Part model, mm, in its own coordinate system. Face numbers are marked on the shaded views. Coordinates: 2 decimals unless noted, no trailing zeros. Loops run counter-clockwise (first coordinate to the right, second up) from the corner with the lowest first, then second, coordinate; pieces in that order, holes last. Notation, with made-up numbers: (69, 88.25) -> (111, 88.25) arc R23 ccw to (111, 100.25) -> close; hole circle Ø2 at (28, -35). An arc over 180 degrees is marked (long way). One line per question, with ' | ' between items. Start each with the question number.
1) Cut at D-D (x = 4.5). List the corners of the cut face in (y, z), plus the area to 3 significant figures.
2) Cut at C-C (x = 28). List the corners of the cut face in (y, z), plus the area to 3 significant figures.
3) Cut at A-A (z = 15). List the corners of the cut face in (x, y).
4) Two-plate mould, pull along X, no slides. Class the marked faces 1, 2, 3 and 4: released by +X, released by -X, zero draft, split by the parting line, or undercut.
5) Cut at B-B (y = -53). List the corners of the cut face in (x, z), plus the area to 3 significant figures.
6) Drop flat-ended pins along their axis: pin 1 (4 mm diameter, centred on x = -6, y = -44.5, fed in from +Z); pin 2 (5 mm diameter, centred on y = -6.5, z = 12, fed in from +X); pin 3 (6 mm diameter, centred on x = -27, y = -35.5, fed in from +Z). Give the stop position or say it passes through.
7) Probe L1, parallel to Y at x = 7, z = 9.75; L2, parallel to Y at x = -9, z = 6.75; L3, parallel to Y at x = -2, z = 18. List the from-to ranges inside material, lowest first. Write a range as from..to.
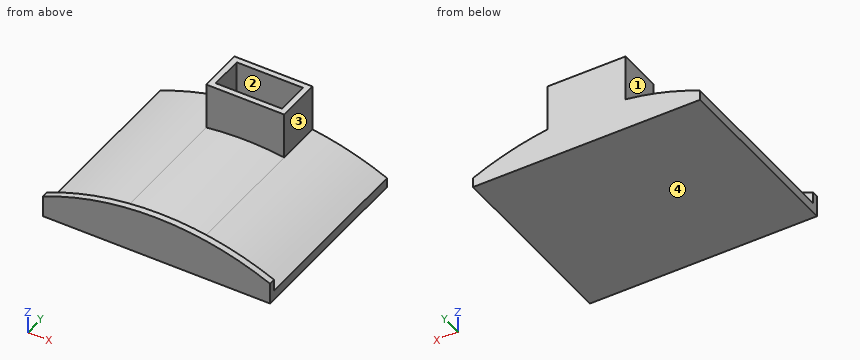
from build123d import *

# Parameters (mm, degrees)
F1_DEPTH = 58
F2_DEPTH = 14
F4_DEPTH = 2
F5_W     = 20.4
F5_H     = 10.4
F6_DEPTH = 22


with BuildPart() as f1:
    # F0 (on Front) → F1 (new body)
    with BuildSketch(Plane.XZ):
        with BuildLine():
            Line((35, -3), (35, 0))
            ThreePointArc((35, 0), (23.7368009031, 4.158739596), (12, 6.6890110215))
            Line((12, 6.6890110215), (12, 0))
            Line((12, 0), (-12, 0))
            Line((-12, 0), (-12, 6.6890110215))
            ThreePointArc((-12, 6.6890110215), (-23.7368009031, 4.158739596), (-35, 0))
            Line((-35, 0), (-35, -3))
            Line((-35, -3), (35, -3))
        make_face()
        with BuildLine():
            Line((12, 0), (12, 6.6890110215))
            ThreePointArc((12, 6.6890110215), (0, 7.5403330759), (-12, 6.6890110215))
            Line((-12, 6.6890110215), (-12, 0))
            Line((-12, 0), (12, 0))
        make_face()
    extrude(amount=F1_DEPTH)

    # F0 (on Front) → F2 (join)
    with BuildSketch(Plane.XZ):
        with BuildLine():
            ThreePointArc((-12, 6.6890110215), (0, 7.5403330759), (12, 6.6890110215))
            Line((12, 6.6890110215), (12, 21))
            Line((12, 21), (-12, 21))
            Line((-12, 21), (-12, 6.6890110215))
        make_face()
    extrude(amount=F2_DEPTH)

    # F3 (on face) → F4 (join)
    with BuildSketch(Plane.XZ.offset(58)):
        with BuildLine():
            Line((35, 0), (35, 3.6027812406))
            ThreePointArc((35, 3.6027812406), (0, 11), (-35, 3.6027812406))
            Line((-35, 3.6027812406), (-35, 0))
            ThreePointArc((-35, 0), (0, 7.5403330759), (35, 0))
        make_face()
    extrude(amount=-F4_DEPTH)

    # F5 (on face) → F6 (cut)
    with BuildSketch(Plane.XY.offset(21)):
        with Locations((0, -7)):
            Rectangle(F5_W, F5_H)
    extrude(amount=-F6_DEPTH, mode=Mode.SUBTRACT)


solid = f1.part
Reported:
1) outline: (-58, -3) -> (0, -3) -> (0, 21) -> (-1.8, 21) -> (-1.8, -1) -> (-12.2, -1) -> (-12.2, 21) -> (-14, 21) -> (-14, 7.42) -> (-56, 7.42) -> (-56, 10.88) -> (-58, 10.88) -> close | area: 573 mm²
2) outline: (-58, -3) -> (0, -3) -> (0, 2.8) -> (-56, 2.8) -> (-56, 6.34) -> (-58, 6.34) -> close | area: 343 mm²
3) outline: (-12, -14) -> (12, -14) -> (12, 0) -> (-12, 0) -> close; hole (-10.2, -12.2) -> (10.2, -12.2) -> (10.2, -1.8) -> (-10.2, -1.8) -> close
4) face 1: released by -X | face 2: undercut | face 3: released by +X | face 4: zero draft
5) outline: (-35, -3) -> (35, -3) -> (35, 0) arc R85 ccw to (-35, 0) -> close | area: 565 mm²
6) pin 1: stops at z = 7.45 | pin 2: stops at x = 12 | pin 3: stops at z = 4.08
7) L1: y = -58..-56, -14..-12.2, -1.8..0 | L2: y = -58..-12.2, -1.8..0 | L3: y = -14..-12.2, -1.8..0
